```python
from build123d import *

# Parameters (mm, degrees)
F1_DEPTH  = 16
F2_W      = 70
F2_H      = 3
F3_DEPTH  = 2
F4_W      = 50
F4_H      = 12
F5_DEPTH  = 2
F6_R      = 2
F9_DEPTH  = 2
F11_DEPTH = 38.001
F13_D     = 4
F14_R     = 3
F14_R_2   = 2
F15_DEPTH = 5
F16_R     = 3


# Not quite as in the source:
# - a pattern or mirror of a feature is missing from the dataset's text; its kind, count and spacing are read off the source's solid


with BuildPart() as f1:
    # F0 (on Front) → F1 (new body)
    with BuildSketch(Plane.XZ):
        with BuildLine():
            ThreePointArc((0, -9), (-9, 0), (0, 9))
            Line((0, 9), (94, 9))
            Line((94, 9), (94, 11))
            Line((94, 11), (0, 11))
            ThreePointArc((0, 11), (-11, 0), (0, -11))
            Line((0, -11), (18.2665281953, -11))
            ThreePointArc((18.2665281953, -11), (20.6244584971, -11.7688756304), (22.0759112253, -13.779917654))
            ThreePointArc((22.0759112253, -13.779917654), (60.9393672504, -57.4049197249), (119.3629664678, -57.8431826489))
            ThreePointArc((119.3629664678, -57.8431826489), (127.4740086729, -57.1014451531), (134.6252638265, -61))
            Line((134.6252638265, -61), (137.2771081943, -61))
            ThreePointArc((137.2771081943, -61), (128.7730913255, -55.3547464626), (118.5862940723, -56))
            ThreePointArc((118.5862940723, -56), (61.4655553189, -55.4468201567), (23.7763203843, -12.5212290284))
            ThreePointArc((23.7763203843, -12.5212290284), (21.9669972314, -9.9754593518), (19, -9))
            Line((19, -9), (0, -9))
        make_face()
    extrude(amount=F1_DEPTH)

    # F2 (on face) → F3 (join)
    with BuildSketch(Plane.XY.offset(11)):
        with Locations((59, -17.5)):
            Rectangle(F2_W, F2_H)
    extrude(amount=-F3_DEPTH)

    # F4 (on face) → F5 (join)
    with BuildSketch(Plane.XZ.offset(19)):
        with Locations((69, 5)):
            Rectangle(F4_W, F4_H)
    extrude(amount=-F5_DEPTH)

    # F6
    f6_edges = [f1.edges().sort_by_distance(p)[0] for p in [
        (59, -19, 11),
        (69, -17, 9),
    ]]
    fillet(f6_edges, radius=F6_R)

    # F7: F1 across plane


with BuildPart() as f1_1:
    add(f1.part)
    add(f1.part.mirror(Plane.XZ))

    # F8 (on face) → F9 (cut)
    with BuildSketch(Plane.XY.offset(11)):
        with BuildLine():
            Line((94, 11.8473697647), (35.7999188125, 11.8473697647))
            ThreePointArc((35.7999188125, 11.8473697647), (21.9261214029, 0.9031688421), (34, -11.9995147554))
            Line((34, -11.9995147554), (94, -11.4599181938))
            Line((94, -11.4599181938), (94, 11.8473697647))
        make_face()
    extrude(amount=-F9_DEPTH, mode=Mode.SUBTRACT)

    # F10 (on face) → F11 (cut, through all)
    with BuildSketch(Plane.XZ.offset(19)):
        with BuildLine():
            ThreePointArc((50, 7), (47, 4), (50, 1))
            Line((50, 1), (70, 1))
            ThreePointArc((70, 1), (73, 4), (70, 7))
            Line((70, 7), (50, 7))
        make_face()
    extrude(amount=-F11_DEPTH, mode=Mode.SUBTRACT)

    # F13 (through all)
    with Locations(Plane.XZ.offset(19)):
        with Locations((80, 5)):
            Hole(F13_D / 2)

    # F14 (on face) → F15 (join)
    with BuildSketch(Plane(origin=(0, -17, 0), x_dir=(-1, 0, 0), z_dir=(0, 1, 0))):
        with Locations((-80, 5)):
            Circle(F14_R)
        with Locations((-80, 5)):
            Circle(F14_R_2, mode=Mode.SUBTRACT)
    f15 = extrude(amount=F15_DEPTH)

    # F15_copies: F15 across plane
    add(f15.mirror(Plane.ZX))

    # F16
    f16_edges = [f1_1.edges().sort_by_distance(p)[0] for p in [
        (94, -18, -1),
        (94, 18, -1),
        (44, 18, -1),
        (44, -18, -1),
    ]]
    fillet(f16_edges, radius=F16_R)


solid = f1_1.part
```
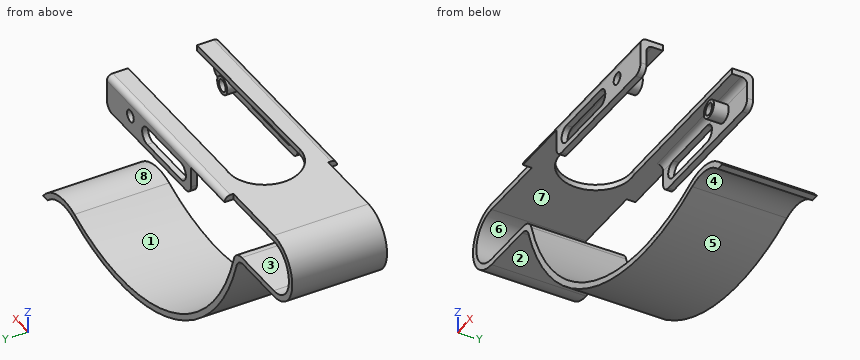
Geometry check sheet. Reference: the model listing, model coordinates, mm. Face numbers are marked on the shaded views. A direction names the side the tool comes from. Give positions to 0.01 mm unless a question says otherwise; leave off trailing zeros. Write each loop counter-clockwise with the first axis right and the second up, starting at its lowest first coordinate (ties: lowest second). Pieces come first, ordered by that corner, then holes. Notation, with made-up numbers: (-20.5, -37) - (3.5, -37) arc R20 ccw to (3.5, -3) - close; hole circle Ø1 at (-7.75, 1). An arc over 180 degrees is marked (long way). Use a Markdown table: item, result.
Q1. Section check B-B, the plane x = 80. Give the number of separate pieces and of enclosed holes in the cut face, then the cut area to 3 significant figures.
Computed:
| item | result |
|---|---|
| separate pieces | 5 |
| enclosed holes | 0 |
| area | 138 mm² |
Q2. Thickness scan on L1, parallel to Y at x = 54, z = 0; L2, parallel to Z at x = 7, y = -3; L3, parallel to Z at x = 78.5, y = -15. Record the ranges inside material, lowest first. Write a range as [from, to].
Computed:
| item | result |
|---|---|
| L1 | y = [-19, -17], [17, 19] |
| L2 | z = [-11, -9], [9, 11] |
| L3 | z = [-62.79, -60.76], [2.4, 3.68], [6.32, 7.6], [9, 11] |
Q3. Section check C-C, the plane y = 9.5. Enter the section's corners in (x, z).
Computed:
| item | result |
|---|---|
| outline | (0, -11) - (18.27, -11) arc R4 cw to (22.08, -13.78) arc R72 ccw to (119.36, -57.84) arc R14 cw to (134.63, -61) - (137.28, -61) arc R16 ccw to (118.59, -56) arc R70 cw to (23.78, -12.52) arc R5 ccw to (19, -9) - (0, -9) arc R9 cw to (0, 9) - (26.56, 9) - (26.56, 11) - (0, 11) arc R11 ccw to start |
Q4. Go/stop test with flat-tipped pins: P1, Ø12, axis at y = -4.5, z = -10.5, coming from the -X side; P2, Ø0.6, axis at x = 65, y = -18.5, coming from the +Z side; P3, Ø10, axis at x = 22.5, y = 10, coming from the -Z side; P4, Ø10, axis at x = 33, z = -44.5, coming from the -Y side. Record where each tip stops, or that it passes through.
Computed:
| item | result |
|---|---|
| P1 | stops at x = -10.04 |
| P2 | stops at z = 10.6 |
| P3 | stops at z = -26.41 |
| P4 | passes through |
Q5. Section check A-A, the plane x = 2. Enter the section's corners in (y, z), then the cut area to 3 significant figures.
Computed:
| item | result |
|---|---|
| outline | (-16, -11) - (16, -11) - (16, -9) - (-16, -9) - close; (-16, 9) - (16, 9) - (16, 11) - (-16, 11) - close |
| area | 128 mm² |
Q6. Draft check along Z on the marked faces 5, 6, 7 and 8. Enter one of: pulls with the +Z half, pulls with the -Z half, needs draft (parallel to the pull), parting line crosses it, or undercut.
Computed:
| item | result |
|---|---|
| face 5 | pulls with the -Z half |
| face 6 | undercut |
| face 7 | undercut |
| face 8 | pulls with the +Z half |
Q7. Set-up check for the marked faces 1, 2, 3 and 4: record each of +Z, -Z, +X, -X, +Y, -Y from which the full face is reachable in a straight line by a thin tool's end or side.
Computed:
| item | result |
|---|---|
| face 1 | +Y, -Y |
| face 2 | -Z, -X, +Y, -Y |
| face 3 | +X, +Y, -Y |
| face 4 | -Z, +Y, -Y |
Q8. Section check D-D, the plane z = -34. Enter the section's corners in (x, y), then the cut area to 3 significant figures.
Computed:
| item | result |
|---|---|
| outline | (32.29, -16) - (34.78, -16) - (34.78, 16) - (32.29, 16) - close |
| area | 79.6 mm² |
